The listing builds one solid part. Answer for the finished solid, in the listing's coordinates (mm). Face numbers are marked on the shaded views. A direction names the side the tool comes from. Give positions to 0.01 mm unless a question says otherwise; leave off trailing zeros. Order: outer loops, then holes, each group sorted by start corner. A loop starts at its lowest first (then second) coordinate and runs counter-clockwise, first axis right, second up. Notation, with made-up numbers: (-6.5, 13.5) - (31.5, 13.5) arc R26 ccw to (31.5, 50.5) - close; hole circle Ø10 at (29, 59.5). An arc over 180 degrees is marked (long way). Answer in a Markdown table with one row per item.
from build123d import *

# Parameters (mm, degrees)
F2_R     = 2
F3_DEPTH = 25


with BuildPart() as f1:
    # F0 (on Front) → F1 (revolve)
    with BuildSketch(Plane.XZ):
        Polygon((0, 18), (0, 0), (8, 0), (8, 4.5), (2.56604, 4.5), (2.56604, 13), (18, 13), (18, 18), align=None)
    revolve(axis=Axis((1.852863, 0, 0), (1, 0, 0)))

    # F2 (on face) → F3 (cut)
    with BuildSketch(Plane.YZ.offset(8)):
        Circle(F2_R)
    extrude(amount=-F3_DEPTH, mode=Mode.SUBTRACT)


solid = f1.part
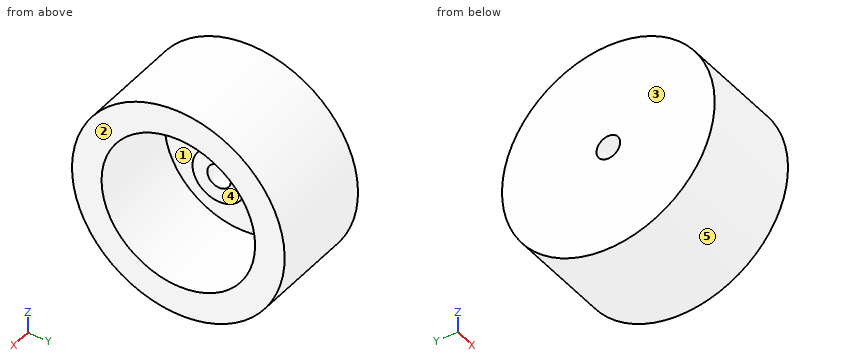
Item 1: Find section C-C on x = 5.25. Write down the section's boundary in (y, z), then the cut area to 3 significant figures.
Answer block:
| item | result |
|---|---|
| outline | circle Ø36 at (0, 0); circle Ø9 at (0, 0); hole circle Ø26 at (0, 0); hole circle Ø4 at (0, 0) |
| area | 538 mm² |
Item 2: Determine the mould class of the marked faces 3, 4 and 5 for opening direction Z: pulls with the +Z half, pulls with the -Z half, needs draft (parallel to the pull), parting line crosses it, or undercut.
Answer block:
| item | result |
|---|---|
| face 3 | needs draft |
| face 4 | undercut |
| face 5 | parting line crosses it |
Item 3: Find section D-D on y = 11. Write down the section's boundary in (x, z), then the cut area to 3 significant figures.
Answer block:
| item | result |
|---|---|
| outline | (0, -14.25) - (18, -14.25) - (18, -6.93) - (2.57, -6.93) - (2.57, 6.93) - (18, 6.93) - (18, 14.25) - (0, 14.25) - close |
| area | 299 mm² |
Item 4: Consider line 1 (Z direction, x = 4.75, y = 0); line 2 (Z direction, x = 8.25, y = 0); line 3 (Z direction, x = 1.5, y = 0). Determine where each line is inside the solid, lowest interval first.
Answer block:
| item | result |
|---|---|
| line 1 | -18 to -13, -4.5 to -2, 2 to 4.5, 13 to 18 |
| line 2 | -18 to -13, 13 to 18 |
| line 3 | -18 to -2, 2 to 18 |
Item 5: Find section A-A on y = 0. Write down the section's boundary in (x, z).
Answer block:
| item | result |
|---|---|
| outline | (0, -18) - (18, -18) - (18, -13) - (2.57, -13) - (2.57, -4.5) - (8, -4.5) - (8, -2) - (0, -2) - close; (0, 2) - (8, 2) - (8, 4.5) - (2.57, 4.5) - (2.57, 13) - (18, 13) - (18, 18) - (0, 18) - close |
Item 6: Each of these flat-tipped pins is pushed along its axis until it touches: P1, Ø6, axis at x = 4.5, y = 13, coming from the +Z side; P2, Ø8, axis at x = 4, z = -7.5, coming from the -Y side; P3, Ø2, axis at x = 2, y = -10.5, coming from the +Z side. Where does it stop, or does it pass through?
Answer block:
| item | result |
|---|---|
| P1 | z = 14.97 |
| P2 | y = -17.66 |
| P3 | z = 15.29 |
Item 7: Which of the six approach directions +Z, -Z, +X, -X, +Y, -Y give full straight-line access (tool end or side, diameter ignored) to the marked faces 1 and 2?
Answer block:
| item | result |
|---|---|
| face 1 | +X |
| face 2 | +Z, -Z, +X, +Y, -Y |
